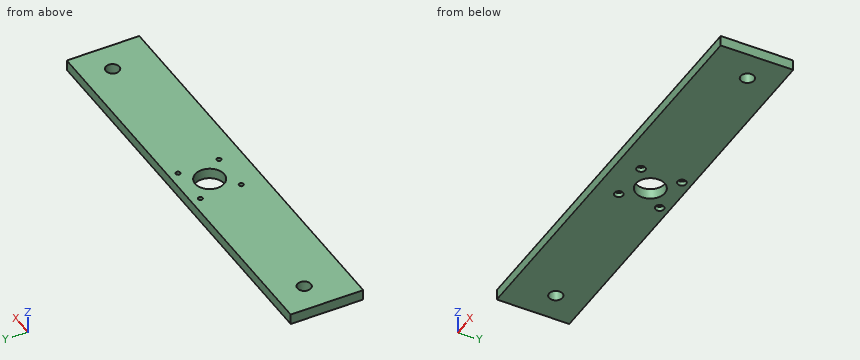
```python
from build123d import *

# Parameters (mm, degrees)
SKETCH1_W                                           = 311.5
SKETCH1_H                                           = 45
BOSS_EXTRUDE1_DEPTH                                 = 4
SKETCH5_R                                           = 11
SKETCH5_R_2                                         = 1.25
CUT_EXTRUDE1_DEPTH                                  = 158.570024116
CBORE_FOR_M3_HEX_SOCKET_HEAD_CAP_SCREW1_D           = 3.4
CBORE_FOR_M3_HEX_SOCKET_HEAD_CAP_SCREW1_CBORE_D     = 6.5
CBORE_FOR_M3_HEX_SOCKET_HEAD_CAP_SCREW1_CBORE_DEPTH = 3.4
F_10_2_10_2_DIAMETER_HOLE1_D                        = 10.2
SKETCH14_W                                          = 311.5
SKETCH14_H                                          = 10
BOSS_EXTRUDE2_DEPTH                                 = 8


with BuildPart() as part:
    # Sketch1 → Boss-Extrude1 (new, symmetric)
    with BuildSketch(Plane.XY):
        Rectangle(SKETCH1_W, SKETCH1_H)
    extrude(amount=BOSS_EXTRUDE1_DEPTH, both=True)

    # Sketch5 → Cut-Extrude1 (cut, through all)
    with BuildSketch(Plane.XY.offset(4)):
        with Locations((-1.75, 0)):
            Circle(SKETCH5_R)
        with Locations((-17.25, 15.5)):
            Circle(SKETCH5_R_2)
        with Locations((13.75, 15.5)):
            Circle(SKETCH5_R_2)
        with Locations((13.75, -15.5)):
            Circle(SKETCH5_R_2)
        with Locations((-17.25, -15.5)):
            Circle(SKETCH5_R_2)
    extrude(amount=-CUT_EXTRUDE1_DEPTH, mode=Mode.SUBTRACT)

    # CBORE for M3 Hex Socket Head Cap Screw1 (through all)
    with Locations(Plane(origin=(0, 0, -4), x_dir=(-1, 0, 0), z_dir=(0, 0, -1))):
        with Locations((-13.75, 15.5), (17.25, 15.5), (17.25, -15.5), (-13.75, -15.5)):
            CounterBoreHole(CBORE_FOR_M3_HEX_SOCKET_HEAD_CAP_SCREW1_D / 2, CBORE_FOR_M3_HEX_SOCKET_HEAD_CAP_SCREW1_CBORE_D / 2, CBORE_FOR_M3_HEX_SOCKET_HEAD_CAP_SCREW1_CBORE_DEPTH)

    # Ø10.2 (10.2) Diameter Hole1 (through all)
    with Locations(Plane.XY.offset(4)):
        with Locations((-133.249958454, 1.369e-06), (133.249998631, 1.369e-06)):
            Hole(F_10_2_10_2_DIAMETER_HOLE1_D / 2)

    # Sketch14 → Boss-Extrude2 (add)
    with BuildSketch(Plane.XY.offset(4)):
        with Locations((0, -27.5)):
            Rectangle(SKETCH14_W, SKETCH14_H)
    extrude(amount=-BOSS_EXTRUDE2_DEPTH)


solid = part.part
```
Here's how the part is built. I have some questions about the finished solid (model axes, mm). Round coordinates to 2 decimals unless told otherwise and drop trailing zeros. Order: outer loops, then holes, each group sorted by start corner. A loop starts at its lowest first (then second) coordinate and runs counter-clockwise, first axis right, second up. Notation, with made-up numbers: M 12,26 L 70,26 A30 cw 70,50 Z; hole C 44.5,48 d4. An arc over 180 degrees is marked long. One line per question, with ' | ' between items.
1) I want a section at A-A, the plane x = -1.75. Write out the boundary of the cut face in (y, z), then the cut area to 3 significant figures.
Working result:
outline: M -32.5,-4 L -11,-4 L -11,4 L -32.5,4 Z; M 11,-4 L 22.5,-4 L 22.5,4 L 11,4 Z | area: 264 mm²
2) For pin 1 Ø9 at (x, y) = (-133.25, 0) entering from -Z; pin 2 Ø5.5 at (x, y) = (13.75, -15.5) entering from -Z, each with a flat end and sliding along its axis, tell me the tip position at first contact or that it passes through.
Working result:
pin 1: through | pin 2: z = -0.6
3) I need wall thicknesses on line 1 along Y through (x, z) = (-17.25, -2.7); line 2 along Y through (x, z) = (13.75, 2.8); line 3 along Y through (x, z) = (-2, 2.5). Which ranges of each line are inside material? Lowest first, please.
Working result:
line 1: -32.5 to -18.75, -12.25 to 12.25, 18.75 to 22.5 | line 2: -32.5 to -17.2, -13.8 to 13.8, 17.2 to 22.5 | line 3: -32.5 to -11, 11 to 22.5
